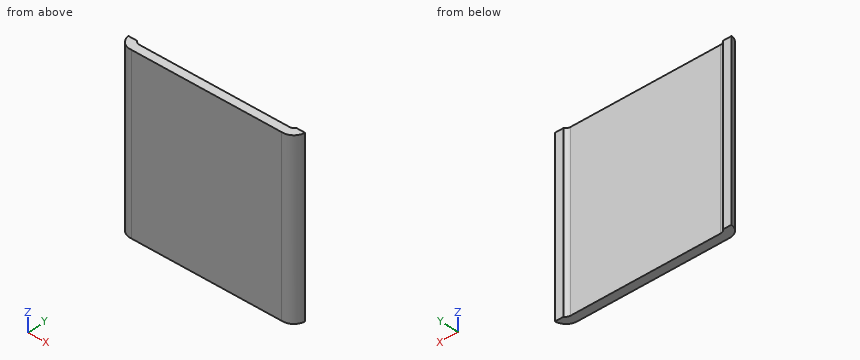
```python
from build123d import *

# Parameters (mm, degrees)
SKETCH1_W           = 350
SKETCH1_H           = 20
BOSS_EXTRUDE1_DEPTH = 400
BOSS_EXTRUDE2_DEPTH = 400


with BuildPart() as part:
    # Sketch1 → Boss-Extrude1 (new body)
    with BuildSketch(Plane.XY):
        Rectangle(SKETCH1_W, SKETCH1_H)
    extrude(amount=BOSS_EXTRUDE1_DEPTH)

    # Sketch2 → Boss-Extrude2 (add)
    with BuildSketch(Plane.XY):
        with BuildLine():
            Line((-175, 10), (-175, -10))
            ThreePointArc((-175, -10), (-195.66613877, -3.40269315), (-205.614305224, 15.875474127))
            Line((-205.614305224, 15.875474127), (-185.614305224, 15.875474127))
            ThreePointArc((-185.614305224, 15.875474127), (-181.041918581, 11.610349673), (-175, 10))
        make_face()
    boss_extrude2 = extrude(amount=BOSS_EXTRUDE2_DEPTH)

    # Mirror1: Boss-Extrude2 across plane
    add(boss_extrude2.mirror(Plane(origin=(0, 0, 0), x_dir=(0, 0, 1), z_dir=(1, 0, 0))))


solid = part.part
```
Geometry check sheet. Reference: the model listing, model coordinates, mm. Give positions to 0.01 mm unless a question says otherwise; leave off trailing zeros. Order: outer loops, then holes, each group sorted by start corner. A loop starts at its lowest first (then second) coordinate and runs counter-clockwise, first axis right, second up.
1. Section check A-A, the plane z = 306.5. Enter the section's corners in (x, y).
2. Section check B-B, the plane x = 20. Enter the section's corners in (y, z).
3. Section check C-C, the plane y = 0.5. Enter the section's corners in (x, z), and give its area (3 significant figures).
4. Gauge pin test, flat ends, axial feed: pin 1 Ø2 at (x, z) = (-151, 122) entering from +Y; pin 2 Ø5 at (y, z) = (-4, 146.5) entering from -X; pin 3 Ø1.5 at (y, z) = (4.5, 72.5) entering from +X. Record the tip position at first contact, or that the pin passes through.
5. Thickness scan on L1, parallel to Y at x = -0.5, z = 182; L2, parallel to X at y = 12.5, z = 139; L3, parallel to X at y = 12.25, z = 103. Record the ranges inside material, lowest first.
Values follow:
1. outline: (-205.61, 15.88) arc R28.34 ccw to (-175, -10) - (175, -10) arc R28.34 ccw to (205.61, 15.88) - (185.61, 15.88) arc R12.89 cw to (175, 10) - (-175, 10) arc R12.89 cw to (-185.61, 15.88) - close
2. outline: (-10, 0) - (10, 0) - (10, 400) - (-10, 400) - close
3. outline: (-199.47, 0) - (199.47, 0) - (199.47, 400) - (-199.47, 400) - close
3. area: 160,000 mm2
4. pin 1: stops at y = 10
4. pin 2: stops at x = -197.7
4. pin 3: stops at x = 202.56
5. L1: y = -10 to 10
5. L2: x = -205.13 to -182.43, 182.43 to 205.13
5. L3: x = -205.07 to -182.08, 182.08 to 205.07
